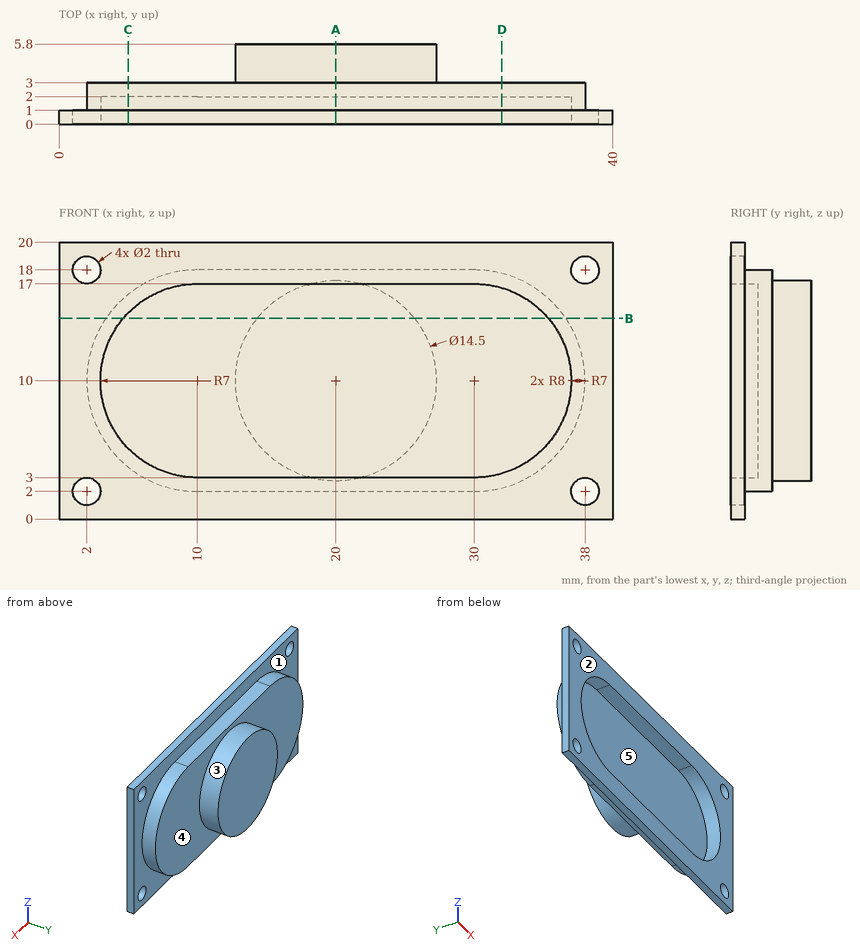
The figure shows three views and two pictorial views of one solid part (mm, origin at its lowest corner). Answer the questions. A direction names the side the tool comes from. Give positions to 0.01 mm unless a question says otherwise; leave off trailing zeros. Order: outer loops, then holes, each group sorted by start corner. A loop starts at its lowest first (then second) coordinate and runs counter-clockwise, first axis right, second up. Notation, with made-up numbers: M 41,60 L 85,60 A17 ccw 85,90 Z; hole C 51.25,-2 d3. An arc over 180 degrees is marked long. Return JSON: item names as keys, results as strings.
1) For a pull along Z with two mould halves and no side action, classify the marked faces 3, 4 and 5 as +Z half, -Z half, draft (parallel to the pull), parting line (faces both ways), or undercut.
Resolved:
{"face 3": "parting line", "face 4": "draft", "face 5": "undercut"}
2) Section A-A, the plane x = 20 is taken. Write down the section's boundary in (y, z), plus the area to 3 significant figures.
Resolved:
{"outline": "M 0,0 L 1,0 L 1,2 L 3,2 L 3,2.75 L 5.8,2.75 L 5.8,17.25 L 3,17.25 L 3,18 L 1,18 L 1,20 L 0,20 L 0,17 L 2,17 L 2,3 L 0,3 Z", "area": "64.6 mm^2"}
3) A tool of negligible diameter and unlimited length cuts with its end or side. For the marked faces 1 and 2, from which of +Z, -Z, +X, -X, +Y, -Y can it reach the whole face along a straight path? Write none if from no direction.
Resolved:
{"face 1": "+Y", "face 2": "+Z, -Z, +X, -X, -Y"}
4) Section B-B, the plane z = 14.5 is taken. Write down the section's boundary in (x, y).
Resolved:
{"outline": "M 0,0 L 4.64,0 L 4.64,2 L 35.36,2 L 35.36,0 L 40,0 L 40,1 L 36.61,1 L 36.61,3 L 25.68,3 L 25.68,5.8 L 14.32,5.8 L 14.32,3 L 3.39,3 L 3.39,1 L 0,1 Z"}
5) Section C-C, the plane x = 5 is taken. Write down the section's boundary in (y, z) (3 decimals), plus the area to 3 significant figures.
Resolved:
{"outline": "M 0,0 L 1,0 L 1,3.755 L 3,3.755 L 3,16.245 L 1,16.245 L 1,20 L 0,20 L 0,14.899 L 2,14.899 L 2,5.101 L 0,5.101 Z", "area": "25.4 mm^2"}
6) Straight lines are drawn through the part: line 1 along Z through (x, y) = (2, 0.2); line 2 along X through (y, z) = (0.7, 18); line 3 along Z through (x, y) = (17, 1.35). For each, find the intervals that lie inside material, in ascending order. Write a range as [from, to].
Resolved:
{"line 1": "[0, 1], [3, 17], [19, 20]", "line 2": "[0, 1], [3, 37], [39, 40]", "line 3": "[2, 3], [17, 18]"}
7) Each of these flat-tipped pins is pushed along its axis until it touches: pin 1 (2 mm diameter, centred on x = 13, y = 2.5, fed in from +Z); pin 2 (1.6 mm diameter, centred on x = 2, z = 2, fed in from -Y); pin 3 (2 mm diameter, centred on x = 16.5, y = 3.5, fed in from -Z); pin 4 (6 mm diameter, centred on x = 7, z = 13, fed in from +Y). Where does it stop, or does it pass through?
Resolved:
{"pin 1": "z = 18", "pin 2": "through", "pin 3": "z = 2", "pin 4": "y = 3"}
8) Section D-D, the plane x = 32 is taken. Write down the section's boundary in (y, z), plus the area to 3 significant figures.
Resolved:
{"outline": "M 0,0 L 1,0 L 1,2.25 L 3,2.25 L 3,17.75 L 1,17.75 L 1,20 L 0,20 L 0,16.71 L 2,16.71 L 2,3.29 L 0,3.29 Z", "area": "24.2 mm^2"}
